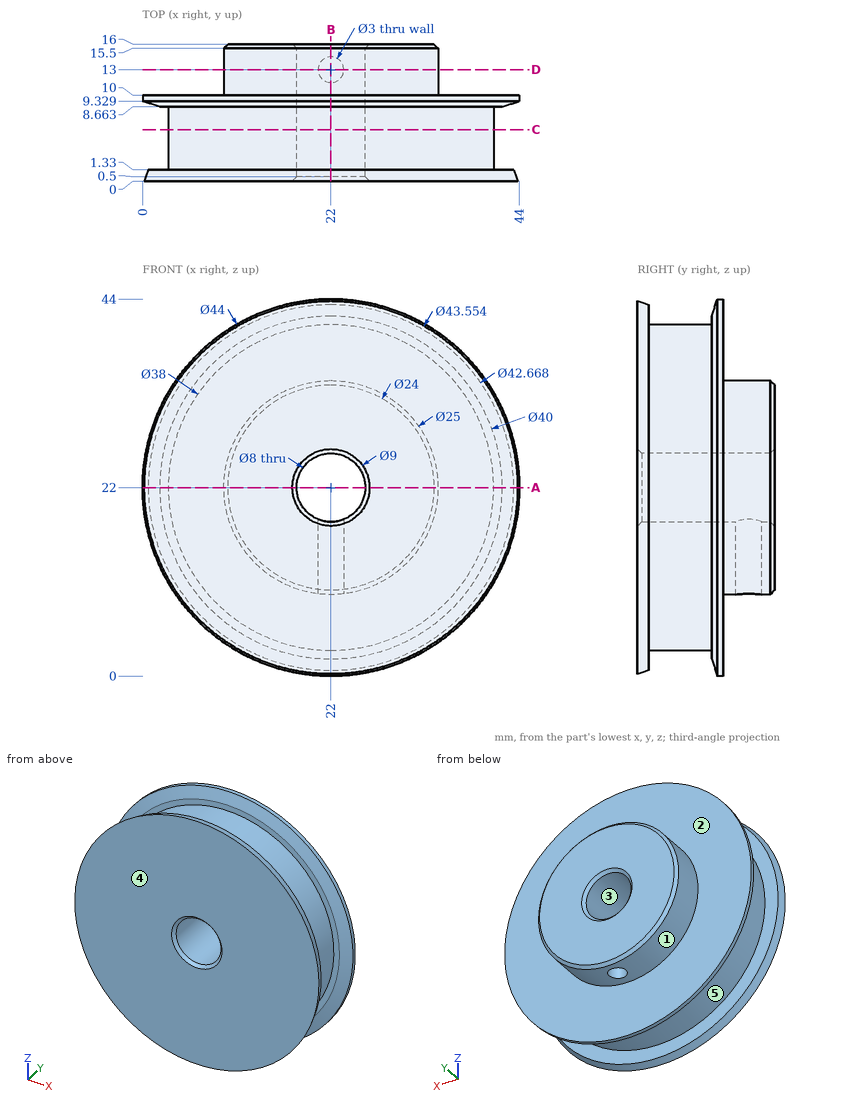
Drawing for the job (mm, zero at the part's lowest x, y, z). A direction names the side the tool comes from. Coordinates: 2 decimals unless noted, no trailing zeros. Loops run counter-clockwise (first coordinate to the right, second up) from the corner with the lowest first, then second, coordinate; pieces in that order, holes last. Notation, with made-up numbers: (85.25, 58.25) - (142.25, 58.25) arc R17 cw to (142.25, 68.25) - close; hole circle Ø3 at (-37.5, 88.5). An arc over 180 degrees is marked (long way). Use CSV: the item, a comma, the result in double quotes. Start each with the question number.
Q1. Probe probe 1 along X at (y, z) = (6, 22); probe 2 along Z at (x, y) = (22, 9.5); probe 3 along X at (y, z) = (11, 22). List the from-to ranges inside material, lowest first. Write a range as from..to.
Q2. Two-plate mould, pull along X, no slides. Class the marked faces 1, 2 and 3: +X half, -X half, draft (parallel to the pull), parting line (faces both ways), or undercut.
Q3. Drop flat-ended pins along their axis: P1, Ø5, axis at x = 22, z = 22, coming from the +Y side; P2, Ø3.5, axis at x = 22, y = 13, coming from the +Z side; P3, Ø2, axis at x = 30.5, z = 35.5, coming from the +Y side; P4, Ø3, axis at x = 35, y = 9.5, coming from the -Z side (1 decimal). Give the stop position or say it passes through.
Q4. Cut at D-D, the plane y = 13. List the corners of the cut face in (x, z).
Q5. Cut at A-A, the plane z = 22. List the corners of the cut face in (x, y).
Q6. Cut at C-C, the plane y = 6. List the corners of the cut face in (x, z), then the cut area to 3 significant figures.
Q7. Cut at B-B, the plane x = 22. State how many separate pieces and enclosed holes the cut face has, then the cut area to 3 significant figures.
Q8. 3-axis set-ups, long thin cutter, end or side, ignore diameter. For the marked faces 4 and 5: which of +Z, -Z, +X, -X, +Y, -Y reach the whole face in a straight line?
Here are the results:
1,probe 1,"3..18, 26..41"
1,probe 2,"0..18, 26..44"
1,probe 3,"9.5..18, 26..34.5"
2,face 1,"parting line"
2,face 2,"draft"
2,face 3,"undercut"
3,P1,"through"
3,P2,"z = 34.5"
3,P3,"y = 10"
3,P4,"z = 3.2"
4,outline,"(20.5, 9.59) - (20.5, 18.29) arc R4 cw (long way) to (23.5, 18.29) - (23.5, 9.59) arc R12.5 ccw (long way) to start"
5,outline,"(0, 9.33) - (2, 8.66) - (3, 8.66) - (3, 1.33) - (0.67, 1.33) - (0.22, 0) - (17.5, 0) - (18, 0.5) - (18, 15.5) - (17.5, 16) - (10, 16) - (9.5, 15.5) - (9.5, 10) - (0, 10) - close; (26, 0.5) - (26.5, 0) - (43.78, 0) - (43.33, 1.33) - (41, 1.33) - (41, 8.66) - (42, 8.66) - (44, 9.33) - (44, 10) - (34.5, 10) - (34.5, 15.5) - (34, 16) - (26.5, 16) - (26, 15.5) - close"
6,outline,"circle Ø38 at (22, 22); hole circle Ø8 at (22, 22)"
6,area,"1,080 mm2"
7,separate pieces,"3"
7,enclosed holes,"0"
7,area,"389 mm2"
8,face 4,"+Z, -Z, +X, -X, -Y"
8,face 5,"none"
